```python
from build123d import *

# Parameters (mm, degrees)
SKETCH1_W           = 60
SKETCH1_H           = 65
BOSS_EXTRUDE1_DEPTH = 20
SKETCH2_R           = 6
CUT_EXTRUDE1_DEPTH  = 21
SKETCH2_3_R         = 2.5
CUT_EXTRUDE2_DEPTH  = 5
SKETCH2_4_R         = 2.5
BOSS_EXTRUDE2_DEPTH = 90
CHAMFER1_SIZE       = 1
CHAMFER2_SIZE       = 3


with BuildPart() as part:
    # Sketch1 → Boss-Extrude1 (new body)
    with BuildSketch(Plane(origin=(0, 0, 0), x_dir=(1, 0, 0), z_dir=(0, 1, 0))):
        with Locations((30, 32.5)):
            Rectangle(SKETCH1_W, SKETCH1_H)
    extrude(amount=BOSS_EXTRUDE1_DEPTH)

    # Sketch2 → Cut-Extrude1 (cut, through all)
    with BuildSketch(Plane(origin=(0, 20, 0), x_dir=(1, 0, 0), z_dir=(0, 1, 0))):
        with Locations((52, 51)):
            Circle(SKETCH2_R)
        with Locations((10, 11)):
            Circle(SKETCH2_R)
    extrude(amount=-CUT_EXTRUDE1_DEPTH, mode=Mode.SUBTRACT)

    # Sketch2<3> → Cut-Extrude2 (cut)
    with BuildSketch(Plane(origin=(0, 20, 0), x_dir=(1, 0, 0), z_dir=(0, 1, 0))):
        with Locations((19.5, 43)):
            Circle(SKETCH2_3_R)
        with Locations((42.5, 20)):
            Circle(SKETCH2_3_R)
    extrude(amount=-CUT_EXTRUDE2_DEPTH, mode=Mode.SUBTRACT)

    # Sketch2<4> → Boss-Extrude2 (add)
    with BuildSketch(Plane(origin=(0, 20, 0), x_dir=(1, 0, 0), z_dir=(0, 1, 0))):
        with Locations((52, 11)):
            Circle(SKETCH2_4_R)
        with Locations((10, 51)):
            Circle(SKETCH2_4_R)
    extrude(amount=-BOSS_EXTRUDE2_DEPTH)

    # Chamfer1
    chamfer1_edges = [part.edges().sort_by_distance(p)[0] for p in [
        (49.5, -70, -11),
        (7.5, -70, -51),
    ]]
    chamfer(chamfer1_edges, length=CHAMFER1_SIZE)

    # Chamfer2
    chamfer2_edges = [part.edges().sort_by_distance(p)[0] for p in [
        (0, 10, -65),
        (60, 10, -65),
        (60, 10, 0),
        (0, 10, 0),
    ]]
    chamfer(chamfer2_edges, length=CHAMFER2_SIZE)


solid = part.part
```
Here's how the part is built. I have some questions about the finished solid (model axes, mm). A direction names the side the tool comes from. Coordinates: 2 decimals unless noted, no trailing zeros. Order: outer loops, then holes, each group sorted by start corner. A loop starts at its lowest first (then second) coordinate and runs counter-clockwise, first axis right, second up.
Item 1: I'm going to push flat-ended pins straight in: pin 1 Ø10 at (y, z) = (-31.5, -9) entering from -X; pin 2 Ø2 at (x, z) = (39, -49) entering from -Y; pin 3 Ø2.5 at (x, z) = (43.5, -21) entering from +Y; pin 4 Ø10 at (x, y) = (46.5, -50) entering from +Z. Where does each tip first touch, or does it pass through?
Response values:
pin 1: stops at x = 49.5
pin 2: stops at y = 0
pin 3: stops at y = 20
pin 4: stops at z = -8.55
Item 2: If we section it at A-A, the plane z = -11: List the corners of the cut face in (x, y) for me, then the cut area to 3 significant figures.
Response values:
outline: (0, 0) - (4, 0) - (4, 20) - (0, 20) - close; (16, 0) - (49.5, 0) - (49.5, -69) - (50.5, -70) - (53.5, -70) - (54.5, -69) - (54.5, 0) - (60, 0) - (60, 20) - (16, 20) - close
area: 1,310 mm2
Item 3: Thinking about a two-plate mould opening in X: for faces 1 (the face through (42, 15, -20)), 2 (the face through (59, 10, -63)), 3 (the face through (30, 10, -65)), which applies, pulls with the +X half, pulls with the -X half, needs draft (parallel to the pull), parting line crosses it, or undercut?
Response values:
face 1: undercut
face 2: pulls with the +X half
face 3: needs draft
Item 4: If we section it at D-D, the plane z = -20: List the corners of the cut face in (x, y) for me, then the cut area to 4 significant figures.
Response values:
outline: (0, 0) - (60, 0) - (60, 20) - (45, 20) - (45, 15) - (40, 15) - (40, 20) - (0, 20) - close
area: 1,175 mm2
Item 5: If we section it at B-B, the plane x = 52: List the corners of the cut face in (y, z) for me, then the cut area to 3 significant figures.
Response values:
outline: (-70, -12.5) - (-69, -13.5) - (0, -13.5) - (0, -45) - (20, -45) - (20, 0) - (0, 0) - (0, -8.5) - (-69, -8.5) - (-70, -9.5) - close; (0, -65) - (20, -65) - (20, -57) - (0, -57) - close
area: 1,410 mm2
Item 6: If we section it at C-C, the plane x = 19.5: List the corners of the cut face in (y, z) for me, then the cut area to 4 significant figures.
Response values:
outline: (0, -65) - (20, -65) - (20, -45.5) - (15, -45.5) - (15, -40.5) - (20, -40.5) - (20, 0) - (0, 0) - close
area: 1,275 mm2
Item 7: I need wall thicknesses on probe 1 along Z at (x, y) = (52, 6.25); probe 2 along X at (y, z) = (17, -43); probe 3 along X at (y, z) = (7, -51). Which ranges of each line are inside material? Lowest first, please.
Response values:
probe 1: z = -65 to -57, -45 to 0
probe 2: x = 0 to 17, 22 to 60
probe 3: x = 0 to 46, 58 to 60
Item 8: Which directions (+Z, -Z, +X, -X, +Y, -Y) give clear straight access to the entire face, cutting with the end or side of a thin tool? Please do faces 4 (the face through (2, 10, -64)), 5 (the face through (54.31, -34.02, -10.04)), 6 (the face through (18, 18, -41)).
Response values:
face 4: -Z, -X, +Y, -Y
face 5: -Y
face 6: +Y
